CAD build for the part. Positions are in the model's coordinates, mm. A direction names the side the tool comes from. Give positions to 0.01 mm unless a question says otherwise; leave off trailing zeros. Loops run counter-clockwise (first coordinate to the right, second up) from the corner with the lowest first, then second, coordinate; pieces in that order, holes last. Notation, with made-up numbers: M -35.75,69 L 13.25,69 A21 ccw 13.25,73 Z; hole C 6,66.25 d11. An arc over 180 degrees is marked long. Answer as CSV lines item,"result".
from build123d import *

# Parameters (mm, degrees)
SKETCH1_W           = 10
SKETCH1_H           = 25
BOSS_EXTRUDE1_DEPTH = 25
CUT_EXTRUDE1_DEPTH  = 25
SKETCH3_W           = 15
SKETCH3_H           = 10
BOSS_EXTRUDE2_DEPTH = 10
CUT_EXTRUDE2_DEPTH  = 10
SKETCH5_W           = 25
SKETCH5_H           = 25
BOSS_EXTRUDE3_DEPTH = 10
CUT_EXTRUDE3_DEPTH  = 25


with BuildPart() as part:
    # Sketch1 → Boss-Extrude1 (new body)
    with BuildSketch(Plane.XY):
        with Locations((5, 12.5)):
            Rectangle(SKETCH1_W, SKETCH1_H)
    extrude(amount=BOSS_EXTRUDE1_DEPTH)

    # Sketch2 → Cut-Extrude1 (cut)
    with BuildSketch(Plane(origin=(0, 25, 0), x_dir=(1, 0, 0), z_dir=(0, 1, 0))):
        Polygon((0, 0), (10, 0), (10, -5), align=None)
        Polygon((0, -25), (10, -20), (10, -25), align=None)
    extrude(amount=-CUT_EXTRUDE1_DEPTH, mode=Mode.SUBTRACT)

    # Sketch3 → Boss-Extrude2 (add)
    with BuildSketch(Plane.ZY):
        with Locations((12.5, 10)):
            Rectangle(SKETCH3_W, SKETCH3_H)
    extrude(amount=BOSS_EXTRUDE2_DEPTH)

    # Sketch4 → Cut-Extrude2 (cut)
    with BuildSketch(Plane.ZY.offset(10)):
        Polygon((20, 15), (12.5, 15), (20, 5), align=None)
        Polygon((5, 15), (5, 5), (12.5, 15), align=None)
    extrude(amount=-CUT_EXTRUDE2_DEPTH, mode=Mode.SUBTRACT)

    # Sketch5 → Boss-Extrude3 (add)
    with BuildSketch(Plane.ZY.offset(10)):
        with Locations((12.5, 12.5)):
            Rectangle(SKETCH5_W, SKETCH5_H)
    extrude(amount=BOSS_EXTRUDE3_DEPTH)

    # Sketch6 → Cut-Extrude3 (cut)
    with BuildSketch(Plane(origin=(0, 25, 0), x_dir=(1, 0, 0), z_dir=(0, 1, 0))):
        Polygon((-10, 0), (-20, 0), (-20, -5), align=None)
        Polygon((-20, -25), (-20, -20), (-10, -25), align=None)
    extrude(amount=-CUT_EXTRUDE3_DEPTH, mode=Mode.SUBTRACT)


solid = part.part
1) Band-saw the part on A-A on y = 21.5. Give the cut face in (x, z), and give its area (3 significant figures).
Answer below:
outline,"M -20,5 L -10,0 L -10,25 L -20,20 Z; M 0,0 L 10,5 L 10,20 L 0,25 Z"
area,"400 mm^2"
2) Band-saw the part on B-B on z = 15.5. Give the cut face in (x, y).
Answer below:
outline,"M -20,0 L -10,0 L -10,5 L 0,5 L 0,0 L 10,0 L 10,25 L 0,25 L 0,11 L -10,11 L -10,25 L -20,25 Z"
3) Mould opens along X. For faces 1 (the face through (-5.07, 9.93, 8.698)), 2 (the face through (-15, 25, 12)), 3 (the face through (-20, 13, 12)) say: +X half, -X half, draft (parallel to the pull), parting line (faces both ways), or undercut.
Answer below:
face 1,"undercut"
face 2,"draft"
face 3,"-X half"
4) Band-saw the part on C-C on y = 6. Give the cut face in (x, z).
Answer below:
outline,"M -20,5 L -10,0 L -10,5.75 L 0,5.75 L 0,0 L 10,5 L 10,20 L 0,25 L 0,19.25 L -10,19.25 L -10,25 L -20,20 Z"
5) Which spindle directions (+Z, -Z, +X, -X, +Y, -Y) get a long thin tool onto all of the face, cutting with end or side? Do faces 4 (the face through (5, 25, 12)), 5 (the face through (0, 15, 12)), 6 (the face through (5.07, 12.675, 2.535)), 7 (the face through (-5.07, 10.07, 16.198)), 8 (the face through (-5, 5, 12)). Say none if no direction does.
Answer below:
face 4,"+Z, -Z, +X, -X, +Y"
face 5,"none"
face 6,"-Z, +X, +Y, -Y"
face 7,"+Z, +Y"
face 8,"+Z, -Z, -Y"
6) Band-saw the part on D-D on x = -3.5. Give the cut face in (y, z), and give its area (3 significant figures).
Answer below:
outline,"M 5,5 L 15,12.5 L 5,20 Z"
area,"75.0 mm^2"
7) Drill centre lines: line 1 (X direction, y = 22, z = 7); line 2 (X direction, y = 22, z = 1); line 3 (Z direction, x = -15.25, y = 14.5) (3 decimals). Where is each one in solid material? Low to high. Write a range as from..to.
Answer below:
line 1,"x = -20..-10, 0..10"
line 2,"x = -12..-10, 0..2"
line 3,"z = 2.625..22.375"
8) Flat gauge pins, fed straight in: pin 1 (8 mm diameter, centred on x = -12, z = 3.5, fed in from -Y); pin 2 (8 mm diameter, centred on x = -10.5, y = 20, fed in from +Z). Where does each tip first touch, or does it go through?
Answer below:
pin 1,"stops at y = 0"
pin 2,"stops at z = 25"
